Answer from the drawing. Dimensions are ordinates in mm from the lowest x, y and z of the part. A direction names the side the tool comes from. Coordinates: 2 decimals unless noted, no trailing zeros. Write each loop counter-clockwise with the first axis right and the second up, starting at its lowest first coordinate (ties: lowest second). Pieces come first, ordered by that corner, then holes.
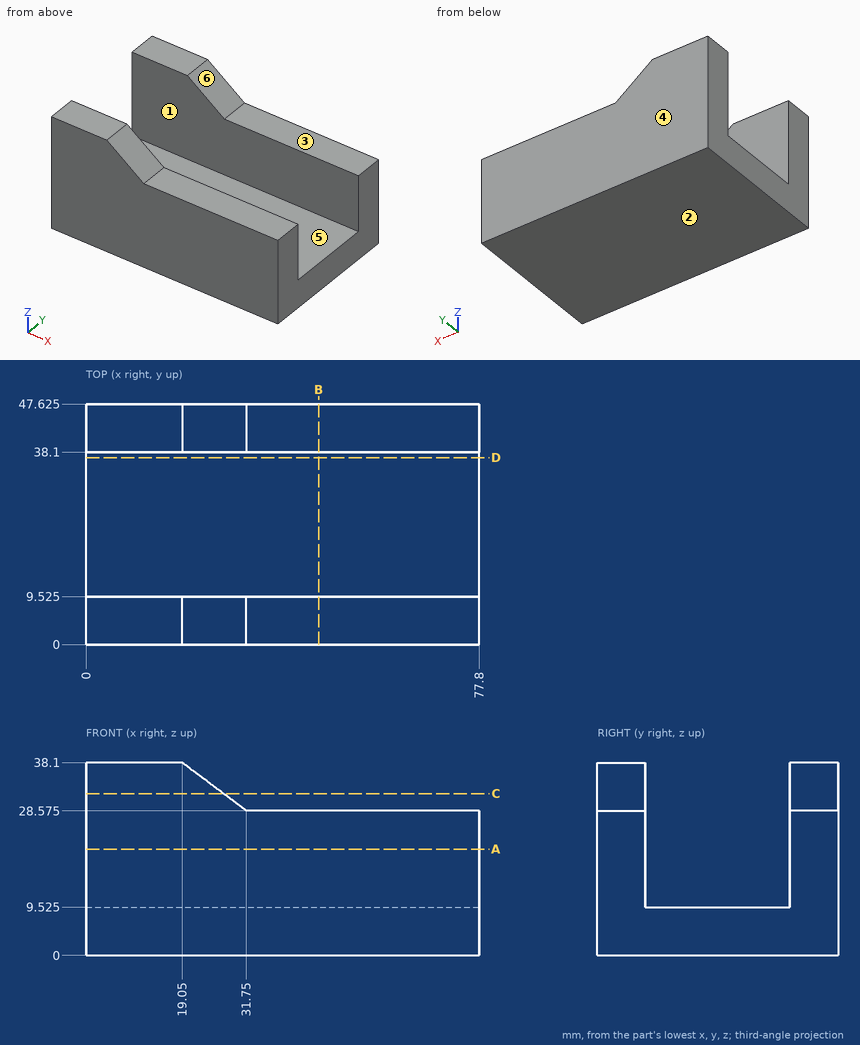
(1) Section A-A, the plane z = 21 is taken. Write down the section's boundary in (x, y) (1 decimal).
(2) Section B-B, the plane x = 46 is taken. Write down the section's boundary in (y, z) (3 decimals).
(3) Section C-C, the plane z = 32 is taken. Write down the section's boundary in (x, y) (1 decimal).
(4) Find the intervals of material crossed by probe 1 along Y at (x, z) = (27.5, 21.5) (3 decimals); probe 2 along Z at (x, y) = (33.5, 33) (3 decimals); probe 3 along Z at (x, y) = (49, 38.5) (3 decimals), in increasing order.
(5) Each of these flat-tipped pins is pushed along its axis until it touches: pin 1 (8 mm diameter, centred on x = 30, z = 30.5, fed in from +Y) (3 decimals); pin 2 (4 mm diameter, centred on x = 21.5, y = 24, fed in from +Z) (3 decimals); pin 3 (3 mm diameter, centred on x = 44, y = 4, fed in from +Z) (3 decimals). Where does it stop, or does it pass through?
(6) Section D-D, the plane y = 37 is taken. Write down the section's boundary in (x, z) (1 decimal).
(7) For a pull along Y with two mould halves and no side action, classify the marked faces 4, 5 and 6 as pulls with the +Y half, pulls with the -Y half, needs draft (parallel to the pull), parting line crosses it, or undercut.
(8) Which of the six approach directions +Z, -Z, +X, -X, +Y, -Y give full straight-line access (tool end or side, diameter ignored) to the marked faces 1, 2 and 3?
Solution:
1. outline: (0, 0) - (77.8, 0) - (77.8, 9.5) - (0, 9.5) - close; (0, 38.1) - (77.8, 38.1) - (77.8, 47.6) - (0, 47.6) - close
2. outline: (0, 0) - (47.625, 0) - (47.625, 28.575) - (38.1, 28.575) - (38.1, 9.525) - (9.525, 9.525) - (9.525, 28.575) - (0, 28.575) - close
3. outline: (0, 0) - (27.2, 0) - (27.2, 9.5) - (0, 9.5) - close; (0, 38.1) - (27.2, 38.1) - (27.2, 47.6) - (0, 47.6) - close
4. probe 1: y = 0 to 9.525, 38.1 to 47.625
4. probe 2: z = 0 to 9.525
4. probe 3: z = 0 to 28.575
5. pin 1: stops at y = 47.625
5. pin 2: stops at z = 9.525
5. pin 3: stops at z = 28.575
6. outline: (0, 0) - (77.8, 0) - (77.8, 9.5) - (0, 9.5) - close
7. face 4: pulls with the +Y half
7. face 5: undercut
7. face 6: needs draft
8. face 1: +Z, +X, -X
8. face 2: -Z, +X, -X, +Y, -Y
8. face 3: +Z, +X, +Y, -Y
